Geometry check sheet. Reference: the model listing, model coordinates, mm. A direction names the side the tool comes from. Round coordinates to 2 decimals unless told otherwise and drop trailing zeros. Write each loop counter-clockwise with the first axis right and the second up, starting at its lowest first coordinate (ties: lowest second). Pieces come first, ordered by that corner, then holes. Notation, with made-up numbers: M 44.5,34 L 65.5,34 A19 cw 65.5,68 Z; hole C 68.5,69.5 d2. An arc over 180 degrees is marked long. One line per item, written item: value. Start each with the question number.
1. Section check B-B (x = 36.5). Record the boundary of the cut face in (y, z) (3 decimals).
2. Section check A-A (x = -12). Record the boundary of the cut face in (y, z) (3 decimals).
3. Section check D-D (y = 0.85). Count the separate pieces of the cut face and the enclosed holes in it, and give its area (3 significant figures).
4. Depth check by flat-ended pin: P1, Ø1.8, axis at x = 45.25, z = -9.16, coming from the +Y side; P2, Ø2.5, axis at x = 0.5, y = 2.5, coming from the +Z side. Enter the tip coordinate at first touch or a pass-through.
5. Scan lines: probe 1 along Z at (x, y) = (51.5, 4.3); probe 2 along X at (y, z) = (1.2, 31.5); probe 3 along X at (y, z) = (4, 10). Record each from-to range of solid material in increasing order. Write a range as [from, to].
6. Release check for a two-part mould opening along Z. For faces 1 (the flat face through (-1, 5, 0)), 2 (the cylindrical face through (10.77, 2.46, 32.61)), 3 (the flat face through (0, 2, 11)) record: pulls with the +Z half, pulls with the -Z half, needs draft (parallel to the pull), parting line crosses it, or undercut.
7. Section check C-C (z = -2.75). Record the boundary of the cut face in (x, y), and give its area (3 significant figures).
8. Access from +Z, -Z, +X, -X, +Y, -Y to the whole of each face (thin tool, end or side, straight path). Record for faces 4 (the cylindrical face through (26.261, 2.465, -8.825)), 5 (the flat face through (8, 2, 23)).
from build123d import *

# Parameters (mm, degrees)
SKETCH_1_W          = 166
SKETCH_1_H          = 70
EXTRUDE_1_DEPTH     = 5
SKETCH_2_R          = 2.025
CUT_EXTRUDE_1_DEPTH = 5
SKETCH_3_R          = 1.525
SKETCH_3_R_2        = 13.45
CUT_EXTRUDE_2_DEPTH = 81.4
SKETCH_5_W          = 16
SKETCH_5_H          = 48
CUT_EXTRUDE_4_DEPTH = 81.4
FILLET_2_R          = 2


with BuildPart() as part:
    # 草图1 → 凸台-拉伸1 (new body)
    with BuildSketch(Plane(origin=(0, 0, 0), x_dir=(1, 0, 0), z_dir=(0, 1, 0))):
        Rectangle(SKETCH_1_W, SKETCH_1_H)
    extrude(amount=EXTRUDE_1_DEPTH)

    # 草图2 → 切除-拉伸1 (cut)
    with BuildSketch(Plane.XZ):
        with Locations(Location((-12, 31, 0), (0, 0, 270))):
            Circle(SKETCH_2_R)
        with Locations(Location((12, 31, 0), (0, 0, 270))):
            Circle(SKETCH_2_R)
        with Locations(Location((0, 6, 0), (0, 0, 270))):
            Circle(SKETCH_2_R)
    extrude(amount=-CUT_EXTRUDE_1_DEPTH, mode=Mode.SUBTRACT)

    # 草图3 → 切除-拉伸2 (cut)
    with BuildSketch(Plane.XZ):
        with Locations(Location((36.5, 23.5, 0), (0, 0, 270))):
            Circle(SKETCH_3_R)
        with Locations(Location((45.25, 21.155444566, 0), (0, 0, 270))):
            Circle(SKETCH_3_R)
        with Locations(Location((51.655444566, 14.75, 0), (0, 0, 270))):
            Circle(SKETCH_3_R)
        with Locations(Location((54, 6, 0), (0, 0, 270))):
            Circle(SKETCH_3_R)
        with Locations(Location((51.655444566, -2.75, 0), (0, 0, 270))):
            Circle(SKETCH_3_R)
        with Locations(Location((45.25, -9.155444566, 0), (0, 0, 270))):
            Circle(SKETCH_3_R)
        with Locations(Location((36.5, -11.5, 0), (0, 0, 270))):
            Circle(SKETCH_3_R)
        with Locations(Location((27.75, -9.155444566, 0), (0, 0, 270))):
            Circle(SKETCH_3_R)
        with Locations(Location((21.344555434, -2.75, 0), (0, 0, 270))):
            Circle(SKETCH_3_R)
        with Locations(Location((19, 6, 0), (0, 0, 270))):
            Circle(SKETCH_3_R)
        with Locations(Location((21.344555434, 14.75, 0), (0, 0, 270))):
            Circle(SKETCH_3_R)
        with Locations(Location((27.75, 21.155444566, 0), (0, 0, 270))):
            Circle(SKETCH_3_R)
        with Locations(Location((36.5, 6, 0), (0, 0, 270))):
            Circle(SKETCH_3_R_2)
    cut_extrude_2 = extrude(amount=-CUT_EXTRUDE_2_DEPTH, mode=Mode.SUBTRACT)

    # 镜向1: 切除-拉伸2 across plane
    add(cut_extrude_2.mirror(Plane(origin=(0, 0, 0), x_dir=(0, 0, 1), z_dir=(1, 0, 0))), mode=Mode.SUBTRACT)

    # 草图5 → 切除-拉伸4 (cut)
    with BuildSketch(Plane.XZ):
        with Locations((0, 35)):
            Rectangle(SKETCH_5_W, SKETCH_5_H)
    extrude(amount=-CUT_EXTRUDE_4_DEPTH, mode=Mode.SUBTRACT)

    # 圆角2
    fillet_2_edges = [part.edges().sort_by_distance(p)[0] for p in [
        (8, 2.5, 35),
        (8, 2.5, 11),
        (-8, 2.5, 35),
        (-8, 2.5, 11),
    ]]
    fillet(fillet_2_edges, radius=FILLET_2_R)


solid = part.part
Result sheet:
1. outline: M 0,-35 L 5,-35 L 5,-13.025 L 0,-13.025 Z; M 0,-9.975 L 5,-9.975 L 5,-7.45 L 0,-7.45 Z; M 0,19.45 L 5,19.45 L 5,21.975 L 0,21.975 Z; M 0,25.025 L 5,25.025 L 5,35 L 0,35 Z
2. outline: M 0,-35 L 5,-35 L 5,28.975 L 0,28.975 Z; M 0,33.025 L 5,33.025 L 5,35 L 0,35 Z
3. separate pieces: 1
3. enclosed holes: 29
3. area: 9,890 mm2
4. P1: passes through
4. P2: stops at z = 11
5. probe 1: z = [-35, -4.27], [-1.23, 13.23], [16.27, 35]
5. probe 2: x = [-83, -13.96], [-10.04, -8], [8, 10.04], [13.96, 83]
5. probe 3: x = [-83, -49.34], [-23.66, 23.66], [49.34, 83]
6. face 1: needs draft
6. face 2: undercut
6. face 3: pulls with the +Z half
7. outline: M -83,0 L -53.18,0 L -53.18,5 L -83,5 Z; M -50.13,0 L -46.71,0 L -46.71,5 L -50.13,5 Z; M -26.29,0 L -22.87,0 L -22.87,5 L -26.29,5 Z; M -19.82,0 L 19.82,0 L 19.82,5 L -19.82,5 Z; M 22.87,0 L 26.29,0 L 26.29,5 L 22.87,5 Z; M 46.71,0 L 50.13,0 L 50.13,5 L 46.71,5 Z; M 53.18,0 L 83,0 L 83,5 L 53.18,5 Z
7. area: 565 mm2
8. face 4: +Y, -Y
8. face 5: +Z, +Y, -Y
